```python
from build123d import *

# Parameters (mm, degrees)
SKETCH1_R           = 4.5
BOSS_EXTRUDE1_DEPTH = 1
SKETCH5_R           = 4.5
CUT_EXTRUDE1_DEPTH  = 1
CUT_EXTRUDE1_DRAFT  = 30
FILLET2_R           = 0.4


with BuildPart() as part:
    # Sketch1 → Boss-Extrude1 (new body)
    with BuildSketch(Plane(origin=(0, 0, 0), x_dir=(1, 0, 0), z_dir=(0, 1, 0))):
        with BuildLine():
            Line((6.5, -2.309401077), (6.5, 2.309401077))
            ThreePointArc((6.5, 2.309401077), (6.165063509, 3.559401077), (5.25, 4.474464586))
            Line((5.25, 4.474464586), (1.25, 6.783865663))
            ThreePointArc((1.25, 6.783865663), (0, 7.118802154), (-1.25, 6.783865663))
            Line((-1.25, 6.783865663), (-5.25, 4.474464586))
            ThreePointArc((-5.25, 4.474464586), (-6.165063509, 3.559401077), (-6.5, 2.309401077))
            Line((-6.5, 2.309401077), (-6.5, -2.309401077))
            ThreePointArc((-6.5, -2.309401077), (-6.165063509, -3.559401077), (-5.25, -4.474464586))
            Line((-5.25, -4.474464586), (-1.25, -6.783865663))
            ThreePointArc((-1.25, -6.783865663), (0, -7.118802154), (1.25, -6.783865663))
            Line((1.25, -6.783865663), (5.25, -4.474464586))
            ThreePointArc((5.25, -4.474464586), (6.165063509, -3.559401077), (6.5, -2.309401077))
        make_face()
        with Locations(Location((0, 0, 0), (0, 0, 270))):
            Circle(SKETCH1_R, mode=Mode.SUBTRACT)
    extrude(amount=BOSS_EXTRUDE1_DEPTH)


with BuildPart() as cut_extrude1_tool:
    # Sketch5 → Cut-Extrude1 (with draft: the straight prism first)
    with BuildSketch(Plane(origin=(0, 1, 0), x_dir=(1, 0, 0), z_dir=(0, 1, 0))):
        Circle(SKETCH5_R)
    extrude(amount=-CUT_EXTRUDE1_DEPTH)
    # Cut-Extrude1: the draft: its side faces are tilted about the plane it starts from
    cut_extrude1_sides = [cut_extrude1_tool.faces().sort_by_distance(p)[0] for p in [
        (-4.5, 0.5, 0),
    ]]
    draft(cut_extrude1_sides, Plane(origin=(0, 1, 0), x_dir=(1, 0, 0), z_dir=(0, 1, 0)), CUT_EXTRUDE1_DRAFT)


with BuildPart() as part_1:
    add(part.part)

    # Cut-Extrude1: cut by cut_extrude1_tool
    add(cut_extrude1_tool.part, mode=Mode.SUBTRACT)

    # Fillet2
    fillet2_edges = [part_1.edges().sort_by_distance(p)[0] for p in [
        (6.5, 0, 0),
        (6.165063509, 0, 3.559401077),
        (3.25, 0, 5.629165125),
        (0, 0, 7.118802154),
        (-3.25, 0, 5.629165125),
        (-6.165063509, 0, 3.559401077),
        (-6.5, 0, 0),
        (-6.165063509, 0, -3.559401077),
        (-3.25, 0, -5.629165125),
        (0, 0, -7.118802154),
        (3.25, 0, -5.629165125),
        (6.165063509, 0, -3.559401077),
    ]]
    fillet(fillet2_edges, radius=FILLET2_R)


solid = part_1.part
```
Build history of the part. All positions in model axes, mm. Round coordinates to 2 decimals unless told otherwise and drop trailing zeros. Write each loop counter-clockwise with the first axis right and the second up, starting at its lowest first coordinate (ties: lowest second). Pieces come first, ordered by that corner, then holes.
1) Band-saw the part on B-B, the plane x = 0. List the corners of the cut face in (y, z), and give its area (3 significant figures).
2) Band-saw the part on A-A, the plane z = 0. List the corners of the cut face in (x, y), and give its area (3 significant figures).
3) Band-saw the part on C-C, the plane y = 0.8. List the corners of the cut face in (x, z).
4) Pin check, flat tip, straight feed: pin 1 (1 mm diameter, centred on x = -4.5, z = -5, fed in from +Y). Stop position of the tip, or through.
5) Drill centre lines: probe 1 along X at (y, z) = (0.3, 4.25); probe 2 along X at (y, z) = (0.9, 3); probe 3 along Z at (x, y) = (1, 0.9). Where is each one in solid material? Low to high.
Ans:
1. outline: (0, -6.72) arc R0.4 ccw to (0.4, -7.12) - (1, -7.12) - (1, -4.5) - (0, -5.08) - close; (0, 5.08) - (1, 4.5) - (1, 7.12) - (0.4, 7.12) arc R0.4 ccw to (0, 6.72) - close
1. area: 4.59 mm2
2. outline: (-6.5, 0.4) arc R0.4 ccw to (-6.1, 0) - (-5.08, 0) - (-4.5, 1) - (-6.5, 1) - close; (4.5, 1) - (5.08, 0) - (6.1, 0) arc R0.4 ccw to (6.5, 0.4) - (6.5, 1) - close
2. area: 3.35 mm2
3. outline: (-6.5, -2.31) arc R2.5 ccw to (-5.25, -4.47) - (-1.25, -6.78) arc R2.5 ccw to (1.25, -6.78) - (5.25, -4.47) arc R2.5 ccw to (6.5, -2.31) - (6.5, 2.31) arc R2.5 ccw to (5.25, 4.47) - (1.25, 6.78) arc R2.5 ccw to (-1.25, 6.78) - (-5.25, 4.47) arc R2.5 ccw to (-6.5, 2.31) - close; hole circle Ø9.23 at (0, 0)
4. pin 1: stops at y = 1
5. probe 1: x = -5.56 to -2.45, 2.45 to 5.56
5. probe 2: x = -6.4 to -3.43, 3.43 to 6.4
5. probe 3: z = -6.91 to -4.45, 4.45 to 6.91
